Input: dimensioned drawing with shaded views. Units: mm. Origin: part minimum x, y, z. Round coordinates to 2 decimals unless told otherwise and drop trailing zeros. Loops run counter-clockwise (first coordinate to the right, second up) from the corner with the lowest first, then second, coordinate; pieces in that order, holes last. Notation, with made-up numbers: (65, -14) - (115, -14) arc R20 cw to (115, 7) - close; hole circle Ø6 at (4, 20). An arc over 180 degrees is marked (long way). Use CSV: the item, a comma, the result in double quotes. Start each with the question number.
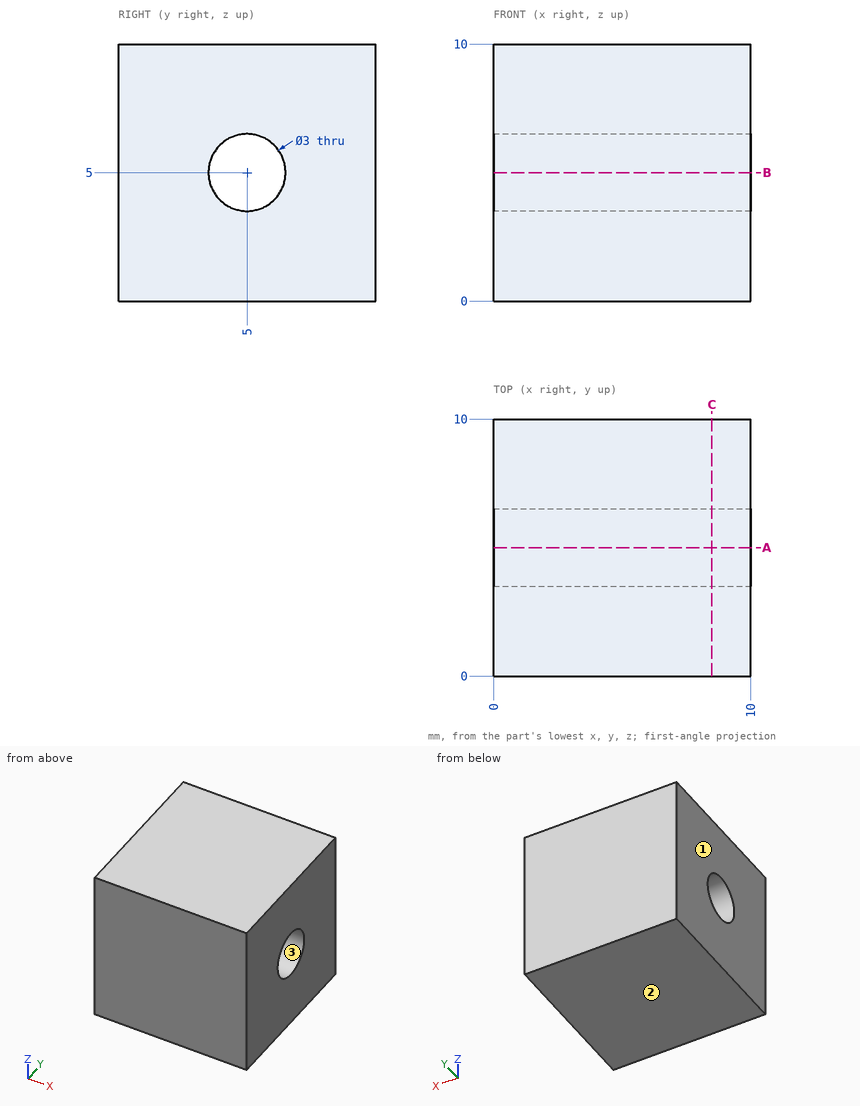
1. Line query: line 1 along Y through (x, z) = (5, 5); line 2 along Y through (x, z) = (8, 4); line 3 along Z through (x, y) = (3.25, 4.25). Output: solid intervals per line, ascending.
2. Section query C-C on x = 8.5. Return the cut outline in (y, z).
3. Contact query for a flat-ended pin moving along its axis: P1, Ø1.8, axis at y = 5, z = 5, coming from the +X side. Output: stop coordinate, or through.
4. Section query A-A on y = 5. Return the cut outline in (x, z).
5. Mould query, pull axis Z, two halves, no side actions, for the marked faces 1, 2 and 3. Classes: +Z half, -Z half, draft (parallel to the pull), parting line (faces both ways), or undercut.
Values:
1,line 1,"y = 0 to 3.5, 6.5 to 10"
1,line 2,"y = 0 to 3.88, 6.12 to 10"
1,line 3,"z = 0 to 3.7, 6.3 to 10"
2,outline,"(0, 0) - (10, 0) - (10, 10) - (0, 10) - close; hole circle Ø3 at (5, 5)"
3,P1,"passes through"
4,outline,"(0, 0) - (10, 0) - (10, 3.5) - (0, 3.5) - close; (0, 6.5) - (10, 6.5) - (10, 10) - (0, 10) - close"
5,face 1,"draft"
5,face 2,"-Z half"
5,face 3,"undercut"
